```python
from build123d import *

# Parameters (mm, degrees)
EXTRUDE_1_DEPTH     = 10
CUT_EXTRUDE_1_REACH = 177.427
SKETCH_2_R          = 2.2
FILLET_1_R          = 0.6
SKETCH_3_W          = 10.144437824
SKETCH_3_H          = 10
EXTRUDE_2_DEPTH     = 15
CUT_EXTRUDE_2_REACH = 164.61
SKETCH_4_R          = 3.8
FILLET_2_R          = 3


with BuildPart() as part:
    # 草图1 → 凸台-拉伸1 (new body)
    with BuildSketch(Plane(origin=(0, 0, 0), x_dir=(1, 0, 0), z_dir=(0, 1, 0))):
        with BuildLine():
            Line((-19, 0), (19, 0))
            Line((19, 0), (44.854614973, 30.81233028))
            ThreePointArc((44.854614973, 30.81233028), (46.529317931, 33.929104052), (46.82231051, 37.455159084))
            Line((46.82231051, 37.455159084), (33.389549678, 146.856216784))
            ThreePointArc((33.389549678, 146.856216784), (34.753999407, 148.533855984), (36.376927445, 147.104765038))
            ThreePointArc((36.376927445, 147.104765038), (36.892496808, 144.296291333), (37.320815542, 141.473193853))
            Line((37.320815542, 141.473193853), (37.815132232, 139.258398169))
            ThreePointArc((37.815132232, 139.258398169), (37.817176658, 139.245056143), (37.817405692, 139.231560332))
            Line((37.817405692, 139.231560332), (37.557917484, 134.104765038))
            ThreePointArc((37.557917484, 134.104765038), (40.754926912, 130.959847465), (43.503129215, 134.503681536))
            Line((43.503129215, 134.503681536), (43.077003941, 137.813685213))
            Line((43.077003941, 137.813685213), (42.807637334, 138.925557366))
            ThreePointArc((42.807637334, 138.925557366), (42.806315787, 138.931905108), (42.80540838, 138.938325149))
            Line((42.80540838, 138.938325149), (42.129277547, 145.175318139))
            Line((42.129277547, 145.175318139), (41.965181023, 146.44996701))
            ThreePointArc((41.965181023, 146.44996701), (43.130662006, 148.010841711), (44.727999785, 146.895858405))
            Line((44.727999785, 146.895858405), (66.016482503, 37.376109146))
            ThreePointArc((66.016482503, 37.376109146), (66.063066684, 33.817543133), (64.860464706, 30.468019192))
            Line((64.860464706, 30.468019192), (38.23055697, -15.656334008))
            ThreePointArc((38.23055697, -15.656334008), (35.050772773, -18.836118205), (30.707106781, -20))
            Line((30.707106781, -20), (5.707106781, -20))
            ThreePointArc((5.707106781, -20), (5.515765065, -19.961939766), (5.353553391, -19.853553391))
            Line((5.353553391, -19.853553391), (5, -19.5))
            Line((5, -19.5), (-5, -19.5))
            Line((-5, -19.5), (-5.353553391, -19.853553391))
            ThreePointArc((-5.353553391, -19.853553391), (-5.515765065, -19.961939766), (-5.707106781, -20))
            Line((-5.707106781, -20), (-25.399802658, -20))
            ThreePointArc((-25.399802658, -20), (-30.087775174, -18.833058003), (-33.681629288, -15.604582738))
            Line((-33.681629288, -15.604582738), (-64.860464706, 30.468019192))
            ThreePointArc((-64.860464706, 30.468019192), (-66.063066684, 33.817543133), (-66.016482503, 37.376109146))
            Line((-66.016482503, 37.376109146), (-46.829620455, 141.890886738))
            ThreePointArc((-46.829620455, 141.890886738), (-43.465252598, 152.148967586), (-37.480163066, 161.13372674))
            ThreePointArc((-37.480163066, 161.13372674), (-33.620696298, 161.680216975), (-32.479267504, 157.953116813))
            ThreePointArc((-32.479267504, 157.953116813), (-35.579400499, 146.14570295), (-34.973851142, 133.953116813))
            Line((-34.973851142, 133.953116813), (-47.176674229, 34.569098196))
            ThreePointArc((-47.176674229, 34.569098196), (-47.109221395, 33.75732882), (-46.723670812, 33.03978429))
            Line((-46.723670812, 33.03978429), (-19, 0))
        make_face()
    extrude(amount=EXTRUDE_1_DEPTH)

    # 草图2 → 切除-拉伸1 (cut, up to next)
    with BuildSketch(Plane(origin=(0, 10, 0), x_dir=(1, 0, 0), z_dir=(0, 1, 0)), mode=Mode.PRIVATE) as cut_extrude_1_sk1:
        with Locations(Location((0, -10, 0), (0, 0, 270))):
            Circle(SKETCH_2_R)
    cut_extrude_1_tool1 = extrude(cut_extrude_1_sk1.sketch, amount=-CUT_EXTRUDE_1_REACH, mode=Mode.PRIVATE) & part.part
    # 草图2 → 切除-拉伸1 (cut, up to next)
    with BuildSketch(Plane(origin=(0, 10, 0), x_dir=(1, 0, 0), z_dir=(0, 1, 0)), mode=Mode.PRIVATE) as cut_extrude_1_sk2:
        with Locations(Location((-26, -10, 0), (0, 0, 270))):
            Circle(SKETCH_2_R)
    cut_extrude_1_tool2 = extrude(cut_extrude_1_sk2.sketch, amount=-CUT_EXTRUDE_1_REACH, mode=Mode.PRIVATE) & part.part
    # 草图2 → 切除-拉伸1 (cut, up to next)
    with BuildSketch(Plane(origin=(0, 10, 0), x_dir=(1, 0, 0), z_dir=(0, 1, 0)), mode=Mode.PRIVATE) as cut_extrude_1_sk3:
        with Locations(Location((26, -10, 0), (0, 0, 270))):
            Circle(SKETCH_2_R)
    cut_extrude_1_tool3 = extrude(cut_extrude_1_sk3.sketch, amount=-CUT_EXTRUDE_1_REACH, mode=Mode.PRIVATE) & part.part
    # 草图2 → 切除-拉伸1 (cut, up to next)
    with BuildSketch(Plane(origin=(0, 10, 0), x_dir=(1, 0, 0), z_dir=(0, 1, 0)), mode=Mode.PRIVATE) as cut_extrude_1_sk4:
        with BuildLine():
            Line((-36.549558395, 121.120011078), (-38.607748185, 104.35740041))
            ThreePointArc((-38.607748185, 104.35740041), (-42.47341142, 116.594845153), (-44.332546284, 129.292956179))
            Line((-44.332546284, 129.292956179), (-43.845113062, 129.987442667))
            ThreePointArc((-43.845113062, 129.987442667), (-43.702378092, 130.509625408), (-43.924830211, 131.003146575))
            Line((-43.924830211, 131.003146575), (-44.447419993, 131.543571067))
            ThreePointArc((-44.447419993, 131.543571067), (-44.482588605, 132.737575539), (-44.499925482, 133.931972015))
            ThreePointArc((-44.499925482, 133.931972015), (-41.418283025, 136.952003662), (-38.505677682, 133.768634142))
            ThreePointArc((-38.505677682, 133.768634142), (-38.556072369, 132.542586282), (-38.556286633, 131.315503182))
            Line((-38.556286633, 131.315503182), (-38.546052546, 131.325051295))
            ThreePointArc((-38.546052546, 131.325051295), (-38.780683801, 130.91622187), (-38.744387532, 130.446247504))
            Line((-38.744387532, 130.446247504), (-38.486748585, 129.793872308))
            ThreePointArc((-38.486748585, 129.793872308), (-37.841140795, 125.384806825), (-36.549558395, 121.120011078))
        make_face()
    cut_extrude_1_tool4 = extrude(cut_extrude_1_sk4.sketch, amount=-CUT_EXTRUDE_1_REACH, mode=Mode.PRIVATE) & part.part
    add(cut_extrude_1_tool1.solids().sort_by_distance((0, 10, 10))[0], mode=Mode.SUBTRACT)
    add(cut_extrude_1_tool2.solids().sort_by_distance((-26, 10, 10))[0], mode=Mode.SUBTRACT)
    add(cut_extrude_1_tool3.solids().sort_by_distance((26, 10, 10))[0], mode=Mode.SUBTRACT)
    add(cut_extrude_1_tool4.solids().sort_by_distance((-40.502089, 10, -123.156617))[0], mode=Mode.SUBTRACT)

    # 圆角1
    fillet_1_edges = [part.edges().sort_by_distance(p)[0] for p in [
        (-36.549558395, 5, -121.120011078),
        (-34.973851142, 5, -133.953116813),
    ]]
    fillet(fillet_1_edges, radius=FILLET_1_R)

    # 草图3 → 凸台-拉伸2 (add)
    with BuildSketch(Plane(origin=(70.613618069, 0, -13.725896909), x_dir=(-0.19080899537654988, 0, -0.9816271834476631), z_dir=(0.9816271834476631, 0, -0.19080899537654988))):
        with Locations((29.616052291, 5)):
            Rectangle(SKETCH_3_W, SKETCH_3_H)
    extrude(amount=EXTRUDE_2_DEPTH)

    # 草图4 → 切除-拉伸2 (cut, up to next)
    with BuildSketch(Plane(origin=(-4.68318419, 0, -24.092894031), x_dir=(0.981627183447663, 0, -0.19080899537654997), z_dir=(0.19080899537654997, 0, 0.981627183447663)), mode=Mode.PRIVATE) as cut_extrude_2_sk1:
        with Locations((79.435271618, 5)):
            Circle(SKETCH_4_R)
    cut_extrude_2_tool1 = extrude(cut_extrude_2_sk1.sketch, amount=-CUT_EXTRUDE_2_REACH, mode=Mode.PRIVATE) & part.part
    add(cut_extrude_2_tool1.solids().sort_by_distance((73.292638, 5, -39.249858))[0], mode=Mode.SUBTRACT)

    # 圆角2
    fillet_2_edges = [part.edges().sort_by_distance(p)[0] for p in [
        (79.687016636, 0, -45.659953836),
        (79.687016636, 10, -45.659953836),
    ]]
    fillet(fillet_2_edges, radius=FILLET_2_R)


solid = part.part
```
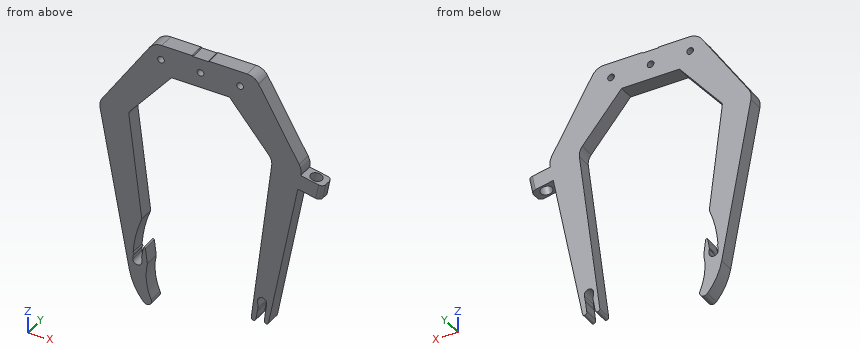
Check sheet for the modelled part. Datum: model origin and axes. Units: mm. Round coordinates to 2 decimals unless told otherwise and drop trailing zeros. Loops run counter-clockwise (first coordinate to the right, second up) from the corner with the lowest first, then second, coordinate; pieces in that order, holes last. Notation, with made-up numbers: (-14.5, -35.75) -> (20.5, -35.75) arc R11 cw to (20.5, -16.75) -> close; hole circle Ø8 at (54.5, -24). An arc over 180 degrees is marked (long way). Write item = value, one per line. Start each with the question number.
1) Thickness scan on probe 1 along X at (y, z) = (1.5, -37.5); probe 2 along X at (y, z) = (3, 10); probe 3 along X at (y, z) = (2.75, -129.5). Record the ranges inside material, lowest first.
2) Sectioned sample at A-A, the plane x = 0. Record the cut outline in (y, z).
3) Sectioned sample at C-C, the plane x = -41.5. Record the cut outline in (y, z).
4) Sectioned sample at B-B, the plane z = -4.5. Record the cut outline in (x, y).
5) Gauge pin test, flat ends, axial feed: pin 1 Ø4 at (y, z) = (4.5, -123.5) entering from -X; pin 2 Ø1.5 at (y, z) = (7.5, -59.5) entering from -X; pin 3 Ø1.5 at (x, y) = (22, 7.5) entering from -Z. Record the tip position at first contact, or that the pin passes through.
6) Sectioned sample at D-D, the plane x = 60.5. Record the cut outline in (y, z), plus the area to 3 significant figures.
Results are:
q1.probe_1 = -65.99 to -46.82, 46.82 to 65.99
q1.probe_2 = -37.47 to -28.2, -23.8 to -2.2, 2.2 to 23.8, 28.2 to 41.5
q1.probe_3 = -49.1 to -44.19, -38.46 to -35.52, 35.52 to 48.11
q2.outline = (0, 0) -> (10, 0) -> (10, 7.8) -> (0, 7.8) -> close; (0, 12.2) -> (10, 12.2) -> (10, 19.5) -> (0, 19.5) -> close
q3.outline = (0, -155.72) -> (10, -155.72) -> (10, -136.95) -> (0, -136.95) -> close; (0, -112.79) -> (10, -112.79) -> (10, -80.8) -> (0, -80.8) -> close; (0, -26.81) -> (10, -26.81) -> (10, 4.05) -> (0, 4.05) -> close
q4.outline = (-47.29, 0) -> (-22.78, 0) -> (-22.78, 10) -> (-47.29, 10) -> close; (22.78, 0) -> (49.87, 0) -> (49.87, 10) -> (22.78, 10) -> close
q5.pin_1 = -50.57
q5.pin_2 = -62.09
q5.pin_3 = -4.47
q6.outline = (0, -65.76) -> (10, -65.76) -> (10, -22.92) -> (0, -22.92) -> close
q6.area = 428 mm^2
